Geometry: final body of the model. Coordinates: model frame, mm. A direction names the side the tool comes from. Give positions to 0.01 mm unless a question says otherwise; leave off trailing zeros. Order: outer loops, then holes, each group sorted by start corner. A loop starts at its lowest first (then second) coordinate and runs counter-clockwise, first axis right, second up. Notation, with made-up numbers: (72.25, -28.5) -> (117.25, -28.5) arc R24 cw to (117.25, 2.5) -> close; hole circle Ø8 at (-27.5, -18.75). An arc over 180 degrees is marked (long way). Answer in a Markdown table with one row per item. Add a question column.
Q1. Contact query for flat-ended pins moving along their axis: P1, Ø1.8, axis at x = 62.87, y = -24.97, coming from the -Z side; P2, Ø1, axis at y = -42, z = 3.5, coming from the -X side. Output: stop coordinate, or through.
Q2. Line query: line 1 along X through (y, z) = (-12.5, 2.6); line 2 along X through (y, z) = (-11, 1.75); line 3 along Y through (x, z) = (80, 1.85). Output: solid intervals per line, ascending. Write a range as from..to.
Q3. Cut plane A-A on x = -50. Return the cut outline in (y, z), and give its area (3 significant figures).
Q4. Set-up query: faces 1 (the face through (116, -21, 2)), 2 (the face through (120, -19, 2)). Return all of +Z, -Z, +X, -X, +Y, -Y with unobstructed straight access to the full face (end or side cutting, diameter ignored); none if empty.
Q5. Cut plane B-B on z = 2.9. Count the separate pieces of the cut face and the enclosed holes in it, and give its area (3 significant figures).
from build123d import *

# Parameters (mm, degrees)
SKETCH_1_R              = 2
EXTRUDE_1_DEPTH         = 5
SKETCH_2_R              = 2.75
SKETCH_2_R_2            = 2
SKETCH_2_R_3            = 2.25
CUT_EXTRUDE_1_DEPTH     = 12
CUT_EXTRUDE_2_OUTLINE_R = 1.5
CUT_EXTRUDE_2_DEPTH     = 5


# Read off the part's stored shape, not the designer's step: 切除-拉伸2
with BuildPart() as part:
    # 草图1 → 凸台-拉伸1 (new body)
    with BuildSketch(Plane.XY):
        with BuildLine():
            Line((-85, -0.312803354), (120, -0.312803354))
            Line((120, -0.312803354), (120, -38.312803354))
            ThreePointArc((120, -38.312803354), (117.071067812, -45.383871166), (110, -48.312803354))
            Line((110, -48.312803354), (-75, -48.312803354))
            ThreePointArc((-75, -48.312803354), (-82.071067812, -45.383871166), (-85, -38.312803354))
            Line((-85, -38.312803354), (-85, -0.312803354))
        make_face()
        with Locations((-80, -11.312803354)):
            Circle(SKETCH_1_R, mode=Mode.SUBTRACT)
        with Locations((0, -11.312803354)):
            Circle(SKETCH_1_R, mode=Mode.SUBTRACT)
        with Locations((80, -11.312803354)):
            Circle(SKETCH_1_R, mode=Mode.SUBTRACT)
        with Locations((75, -36.812803354)):
            Circle(SKETCH_1_R, mode=Mode.SUBTRACT)
        with Locations(Location((-75, -30.812803354, 0), (0, 0, 180))):
            Circle(SKETCH_1_R, mode=Mode.SUBTRACT)
        with Locations((25, -36.812803354)):
            Circle(SKETCH_1_R, mode=Mode.SUBTRACT)
    extrude(amount=EXTRUDE_1_DEPTH)

    # 草图2 → 切除-拉伸1 (cut)
    with BuildSketch(Plane.XY):
        with Locations(Location((-43.5, -18.312803354, 0), (0, 0, 180))):
            Circle(SKETCH_2_R)
        with Locations(Location((107.5, -37.812803354, 0), (0, 0, 180))):
            Circle(SKETCH_2_R_2)
        with Locations(Location((112.5, -44.812803354, 0), (0, 0, 180))):
            Circle(SKETCH_2_R_2)
        with Locations(Location((-50, -12.5, 0), (0, 0, 180))):
            Circle(SKETCH_2_R_3)
        with Locations(Location((-10, -12.5, 0), (0, 0, 180))):
            Circle(SKETCH_2_R_3)
        with Locations(Location((-50, -37.5, 0), (0, 0, 180))):
            Circle(SKETCH_2_R_3)
        with Locations(Location((-10, -37.5, 0), (0, 0, 180))):
            Circle(SKETCH_2_R_3)
        with BuildLine():
            Line((108, -15.312803354), (112, -15.312803354))
            ThreePointArc((112, -15.312803354), (114.828427125, -16.48437623), (116, -19.312803354))
            Line((116, -19.312803354), (116, -23.312803354))
            ThreePointArc((116, -23.312803354), (114.828427125, -26.141230479), (112, -27.312803354))
            Line((112, -27.312803354), (108, -27.312803354))
            ThreePointArc((108, -27.312803354), (105.171572875, -26.141230479), (104, -23.312803354))
            Line((104, -23.312803354), (104, -19.312803354))
            ThreePointArc((104, -19.312803354), (105.171572875, -16.48437623), (108, -15.312803354))
        make_face()
    extrude(amount=CUT_EXTRUDE_1_DEPTH, mode=Mode.SUBTRACT)

    # 切除-拉伸2 outline → 切除-拉伸2 (cut)
    with BuildSketch(Plane.XY):
        with Locations((100.870628671, -24.974954548)):
            Circle(CUT_EXTRUDE_2_OUTLINE_R)
        with Locations((90.870628671, -16.974954548)):
            Circle(CUT_EXTRUDE_2_OUTLINE_R)
        with Locations((81.870628671, -24.974954548)):
            Circle(CUT_EXTRUDE_2_OUTLINE_R)
        with Locations((71.870628671, -16.974954548)):
            Circle(CUT_EXTRUDE_2_OUTLINE_R)
        with Locations((62.870628671, -24.974954548)):
            Circle(CUT_EXTRUDE_2_OUTLINE_R)
        with Locations((52.870628671, -16.974954548)):
            Circle(CUT_EXTRUDE_2_OUTLINE_R)
        with Locations((43.870628671, -24.974954548)):
            Circle(CUT_EXTRUDE_2_OUTLINE_R)
        with Locations((33.870628671, -16.974954548)):
            Circle(CUT_EXTRUDE_2_OUTLINE_R)
        with Locations((24.870628671, -24.974954548)):
            Circle(CUT_EXTRUDE_2_OUTLINE_R)
        with Locations((14.870628671, -16.974954548)):
            Circle(CUT_EXTRUDE_2_OUTLINE_R)
        with Locations((5.870628671, -24.974954548)):
            Circle(CUT_EXTRUDE_2_OUTLINE_R)
        with Locations((-4.129371329, -16.974954548)):
            Circle(CUT_EXTRUDE_2_OUTLINE_R)
    extrude(amount=CUT_EXTRUDE_2_DEPTH, mode=Mode.SUBTRACT)


solid = part.part
Completed:
| question | item | result |
|---|---|---|
| 1 | P1 | passes through |
| 1 | P2 | stops at x = -84.48 |
| 2 | line 1 | x = -85..-81.61, -78.39..-52.25, -47.75..-12.25, -7.75..-1.61, 1.61..78.39, 81.61..120 |
| 2 | line 2 | x = -85..-81.98, -78.02..-51.68, -48.32..-11.68, -8.32..-1.98, 1.98..78.02, 81.98..120 |
| 2 | line 3 | y = -48.31..-13.31, -9.31..-0.31 |
| 3 | outline | (-48.31, 0) -> (-39.75, 0) -> (-39.75, 5) -> (-48.31, 5) -> close; (-35.25, 0) -> (-14.75, 0) -> (-14.75, 5) -> (-35.25, 5) -> close; (-10.25, 0) -> (-0.31, 0) -> (-0.31, 5) -> (-10.25, 5) -> close |
| 3 | area | 195 mm² |
| 4 | face 1 | +Z, -Z |
| 4 | face 2 | +Z, -Z, +X, +Y, -Y |
| 5 | separate pieces | 1 |
| 5 | enclosed holes | 26 |
| 5 | area | 9,390 mm² |
